The model under review builds one solid part; all positions refer to its coordinate system, in mm. A direction names the side the tool comes from. Round coordinates to 2 decimals unless told otherwise and drop trailing zeros. Write each loop counter-clockwise with the first axis right and the second up, starting at its lowest first coordinate (ties: lowest second). Pieces come first, ordered by that corner, then holes. Notation, with made-up numbers: (62.25, 34.25) - (103.25, 34.25) arc R23 ccw to (103.25, 52.25) - close; hole circle Ø10 at (17.5, -21.5). An arc over 180 degrees is marked (long way). Return JSON: item names as keys, results as strings.
from build123d import *

# Parameters (mm, degrees)
EXTRUDE_1_DEPTH             = 10
FILLET_1_R                  = 0.3
FILLET_2_R                  = 2
HOLE_WIZARD_M51_D           = 4.2
HOLE_WIZARD_M51_CSINK_D     = 5.2
HOLE_WIZARD_M51_CSINK_ANGLE = 90


with BuildPart() as part:
    # Эскиз1 → Бобышка-Вытянуть1 (new body, symmetric)
    with BuildSketch(Plane.XY):
        with BuildLine():
            Line((-4, 0), (4, 0))
            Line((4, 0), (4, -0.8))
            Line((4, -0.8), (6, -0.8))
            Line((6, -0.8), (6, -1.6))
            ThreePointArc((6, -1.6), (4.120585945, -4.832650297), (1.5, -7.5))
            Line((1.5, -7.5), (-1.5, -7.5))
            ThreePointArc((-1.5, -7.5), (-4.120585945, -4.832650297), (-6, -1.6))
            Line((-6, -1.6), (-6, -0.8))
            Line((-6, -0.8), (-4, -0.8))
            Line((-4, -0.8), (-4, 0))
        make_face()
    extrude(amount=EXTRUDE_1_DEPTH, both=True)

    # Скругление1
    fillet_1_edges = [part.edges().sort_by_distance(p)[0] for p in [
        (6, -0.8, 0),
        (6, -1.6, 0),
        (-6, -1.6, 0),
        (-6, -0.8, 0),
        (-4, 0, 0),
        (4, 0, 0),
    ]]
    fillet(fillet_1_edges, radius=FILLET_1_R)

    # Скругление2
    fillet_2_edges = [part.edges().sort_by_distance(p)[0] for p in [
        (1.5, -7.5, 0),
        (-1.5, -7.5, 0),
    ]]
    fillet(fillet_2_edges, radius=FILLET_2_R)

    # Отверстие обработанное метчиком M51 (through all)
    with Locations(Plane(origin=(0, 0, 0), x_dir=(1, 0, 0), z_dir=(0, 1, 0))):
        with Locations((0, -4)):
            CounterSinkHole(HOLE_WIZARD_M51_D / 2, HOLE_WIZARD_M51_CSINK_D / 2, counter_sink_angle=HOLE_WIZARD_M51_CSINK_ANGLE)

    # Эскиз5 → Повернуть1 (revolve)
    with BuildSketch(Plane(origin=(0, 0, 0), x_dir=(0, 0, -1), z_dir=(1, 0, 0))):
        with BuildLine():
            Line((6, -4.3), (6, -8.3))
            ThreePointArc((6, -8.3), (4, -6.3), (6, -4.3))
        make_face()
    revolve(axis=Axis((0, -4.3, -6), (0, -1, 0)))


solid = part.part
(1) For faces 1 (the flat face through (0, -7.5, 8)), 2 (the flat face through (5, -0.8, 0)), 3 (the cylindrical face through (-1.49, -7.37, -3.15)), 4 (the cylindrical face through (1.49, -7.37, -3.15)), 5 (the cylindrical face through (-1.49, -7.37, 7.67)), list the 3-axis set-ups (+Z, -Z, +X, -X, +Y, -Y) from which the entire face can be reached by the end or side of a thin tool; tool diameter is ignored.
Filled in:
{"face 1": "+Z, +X, -X, -Y", "face 2": "+Z, -Z, +X, +Y", "face 3": "-X, -Y", "face 4": "+X, -Y", "face 5": "+Z, -X, -Y"}
(2) Add section A-A (x = 0). Write out the cut boundary in (y, z), plus the area to 3 significant figures.
Filled in:
{"outline": "(-7.5, -10) - (0, -10) - (0, 1.4) - (-0.5, 1.9) - (-7.5, 1.9) - (-7.5, -4.4) arc R2 ccw to (-7.5, -7.6) - close; (-7.5, 6.1) - (-0.5, 6.1) - (0, 6.6) - (0, 10) - (-7.5, 10) - close", "area": "120 mm2"}
(3) Wall thickness on line 1 (Z direction, x = 0, y = -5); line 2 (Y direction, x = 0, z = 9); line 3 (X direction, y = -5, z = 5): over which ranges is each line inside the solid? List them lowest first.
Filled in:
{"line 1": "z = -10 to 1.9, 6.1 to 10", "line 2": "y = -7.5 to 0", "line 3": "x = -3.99 to -1.85, 1.85 to 3.99"}
(4) Mouldability with a two-part tool opening along Z and no side actions: class faces 6 (the flat face through (0, -7.5, -1)), 7 (the flat face through (0, -3, -10)), 8 (the cylindrical face through (2.1, -4.05, 3.91)), 9 (the flat face through (0, -3, 10)) as released by +Z, released by -Z, zero draft, split by the parting line, or undercut.
Filled in:
{"face 6": "zero draft", "face 7": "released by -Z", "face 8": "undercut", "face 9": "released by +Z"}
(5) Add section D-D (z = -6.25). Write out the cut boundary in (x, y).
Filled in:
{"outline": "(-6, -1.54) arc R0.3 ccw to (-5.98, -1.66) arc R15 ccw to (-2.1, -7) arc R2 ccw to (-1.74, -7.25) arc R1.98 ccw to (1.74, -7.25) arc R2 ccw to (2.1, -7) arc R15 ccw to (5.98, -1.66) arc R0.3 ccw to (6, -1.54) - (6, -1.1) arc R0.3 ccw to (5.7, -0.8) - (4, -0.8) - (4, -0.3) arc R0.3 ccw to (3.7, 0) - (-3.7, 0) arc R0.3 ccw to (-4, -0.3) - (-4, -0.8) - (-5.7, -0.8) arc R0.3 ccw to (-6, -1.1) - close"}
(6) Add section C-C (y = -6.5). Write out the cut boundary in (x, z), plus the area to 3 significant figures.
Filled in:
{"outline": "(-2.64, -10) - (2.64, -10) - (2.64, 10) - (-2.64, 10) - close; hole circle Ø4.2 at (0, 4)", "area": "91.8 mm2"}
(7) Add section B-B (z = 0). Write out the cut boundary in (x, y).
Filled in:
{"outline": "(-6, -1.54) arc R0.3 ccw to (-5.98, -1.66) arc R15 ccw to (-2.1, -7) arc R2 ccw to (-0.78, -7.5) - (0.78, -7.5) arc R2 ccw to (2.1, -7) arc R15 ccw to (5.98, -1.66) arc R0.3 ccw to (6, -1.54) - (6, -1.1) arc R0.3 ccw to (5.7, -0.8) - (4, -0.8) - (4, -0.3) arc R0.3 ccw to (3.7, 0) - (-3.7, 0) arc R0.3 ccw to (-4, -0.3) - (-4, -0.8) - (-5.7, -0.8) arc R0.3 ccw to (-6, -1.1) - close"}
(8) Clearance check with flat-ended pins moving along their axes: pin 1 Ø0.5 at (x, z) = (0, 7.5) entering from -Y; pin 2 Ø3 at (x, z) = (-3.5, -1.5) entering from -Y; pin 3 Ø1.9 at (x, z) = (-4.5, -2.5) entering from +Y; pin 4 Ø0.8 at (x, z) = (4.5, 1.5) entering from +Y. State where each tip first meets the part, or that it passes through.
Filled in:
{"pin 1": "stops at y = -7.5", "pin 2": "stops at y = -7.08", "pin 3": "stops at y = 0", "pin 4": "stops at y = -0.8"}
